Source: CAD feature listing. Evaluate the final solid. Frame: model axes, mm. Give positions to 0.01 mm unless a question says otherwise; leave off trailing zeros. Order: outer loops, then holes, each group sorted by start corner. A loop starts at its lowest first (then second) coordinate and runs counter-clockwise, first axis right, second up. Notation, with made-up numbers: M 56.5,50 L 95.5,50 A16 cw 95.5,66 Z; hole C -34,66.25 d2. An arc over 180 degrees is marked long. Answer as a JSON object with one key per item and string values. Group by question number.
1. Section query C-C (y = 25). Output: boundary loops of the cut face in (x, z).
2. Section query D-D (z = 44.5). Output: boundary loops of the cut face in (x, y), plus the area to 3 significant figures.
3. Section query A-A (z = 29). Output: boundary loops of the cut face in (x, y), plus the area to 3 significant figures.
4. Section query B-B (x = 23). Output: boundary loops of the cut face in (y, z).
5. Material intervals for L1, parallel to Y at x = 4, z = 34.5; L2, parallel to X at y = 22, z = 47; L3, parallel to X at y = 11, z = 27.5, sorted ascending. Write a range as [from, to].
from build123d import *

# Parameters (mm, degrees)
ESBO_O1_W       = 100
ESBO_O1_H       = 100
EXTRUS_O1_DEPTH = 50


with BuildPart() as part:
    # Esboço1 → Extrusão1 (new body)
    with BuildSketch(Plane.XY):
        Rectangle(ESBO_O1_W, ESBO_O1_H)
    extrude(amount=EXTRUS_O1_DEPTH)

    # Esboço2 → Corte-Revolução1 (revolve, cut)
    with BuildSketch(Plane.XY.offset(50)):
        with BuildLine():
            Line((-27.945356346, 0), (27.945356346, 0))
            ThreePointArc((27.945356346, 0), (0, 27.945356346), (-27.945356346, 0))
        make_face()
    revolve(axis=Axis((-27.945356346, 0, 50), (1, 0, 0)), mode=Mode.SUBTRACT)


solid = part.part
Answer sheet:
{
 "1": {"outline": "M -50,0 L 50,0 L 50,50 L 12.49,50 A12.49 cw -12.49,50 L -50,50 Z"},
 "2": {"outline": "M -50,-50 L 50,-50 L 50,50 L -50,50 Z; hole C 0,0 d54.8", "area": "7,640 mm^2"},
 "3": {"outline": "M -50,-50 L 50,-50 L 50,50 L -50,50 Z; hole C 0,0 d36.88", "area": "8,930 mm^2"},
 "4": {"outline": "M -50,0 L 50,0 L 50,50 L 15.87,50 A15.87 cw -15.87,50 L -50,50 Z"},
 "5": {"L1": "[-50, -22.91], [22.91, 50]", "L2": "[-50, -16.97], [16.97, 50]", "L3": "[-50, -12.4], [12.4, 50]"}
}
